Answer from the drawing. Dimensions are ordinates in mm from the lowest x, y and z of the part. Coordinates: 2 decimals unless noted, no trailing zeros. Write each loop counter-clockwise with the first axis right and the second up, starting at its lowest first coordinate (ties: lowest second). Pieces come first, ordered by that corner, then holes. Notation, with made-up numbers: (55.5, -26) -> (90.5, -26) arc R10 ccw to (90.5, -7) -> close; hole circle Ø10 at (-19.75, 89.5). An arc over 180 degrees is marked (long way). Answer as a JSON object with one key per item and string values. Group by question number.
(1) Straight lines are drawn through the part: L1, parallel to Z at x = 17.56, y = 0.9 (3 decimals); L2, parallel to X at y = 1.95, z = 7.5; L3, parallel to Z at x = 27.5, y = 0.45. For each, find the intervals that lie inside material, in ascending order.
(2) A flat-ended cylindrical pin translates along its axis: P1, Ø1.3, axis at x = 20, y = 1, coming from the -Z side. Find the tip coordinate at first contact, or state that the pin passes through.
(3) Find section B-B (x = 6.5). Give the vertices of the cut face in (y, z).
(4) Find section C-C (y = 1.05). Give the vertices of the cut face in (x, z) (3 decimals).
(5) Find section A-A (x = 17.56). Give the vertices of the cut face in (y, z) (3 decimals), then the cut area to 3 significant figures.
(6) For a pull along Z with two mould halves and no side action, classify the marked faces 1, 2 and 3 as +Z half, -Z half, draft (parallel to the pull), parting line (faces both ways), or undercut.
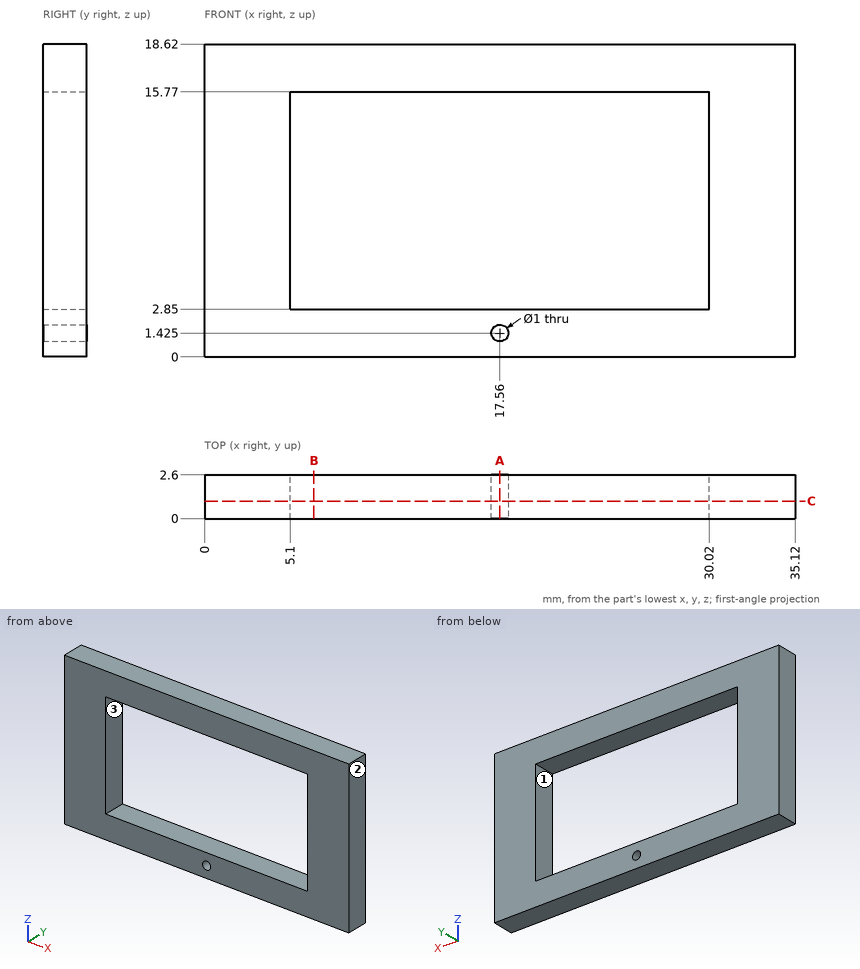
Results below:
{
 "1": {"L1": "z = 0 to 0.925, 1.925 to 2.85, 15.77 to 18.62", "L2": "x = 0 to 5.1, 30.02 to 35.12", "L3": "z = 0 to 2.85, 15.77 to 18.62"},
 "2": {"P1": "stops at z = 0"},
 "3": {"outline": "(0, 0) -> (2.6, 0) -> (2.6, 2.85) -> (0, 2.85) -> close; (0, 15.77) -> (2.6, 15.77) -> (2.6, 18.62) -> (0, 18.62) -> close"},
 "4": {"outline": "(0, 0) -> (35.12, 0) -> (35.12, 18.62) -> (0, 18.62) -> close; hole (5.1, 2.85) -> (30.02, 2.85) -> (30.02, 15.77) -> (5.1, 15.77) -> close; hole circle Ø1 at (17.56, 1.425)"},
 "5": {"outline": "(0, 0) -> (2.6, 0) -> (2.6, 0.925) -> (0, 0.925) -> close; (0, 1.925) -> (2.6, 1.925) -> (2.6, 2.85) -> (0, 2.85) -> close; (0, 15.77) -> (2.6, 15.77) -> (2.6, 18.62) -> (0, 18.62) -> close", "area": "12.2 mm2"},
 "6": {"face 1": "undercut", "face 2": "draft", "face 3": "undercut"}
}
